Verification items for the finished model (mm, model axes). Face numbers are marked on the shaded views. Give positions to 0.01 mm unless a question says otherwise; leave off trailing zeros. Write each loop counter-clockwise with the first axis right and the second up, starting at its lowest first coordinate (ties: lowest second). Pieces come first, ordered by that corner, then holes. Notation, with made-up numbers: (16.25, 54) - (47.25, 54) arc R11 cw to (47.25, 63) - close; hole circle Ø3 at (-29.75, 48.25). An arc over 180 degrees is marked (long way). Answer as a JSON object with one key per item and string values. Group by question number.
Item 1: Sectioned sample at B-B, the plane x = 670. Record the boundary of the cut face in (y, z).
Item 2: Draft check along X on the marked faces 1 and 2. Enter one of: +X half, -X half, draft (parallel to the pull), parting line (faces both ways), or undercut.
Item 3: Scan lines: line 1 along Y through (x, z) = (808.5, 72.5); line 2 along X through (y, z) = (497, 73); line 3 along Z through (x, y) = (926.5, 1291.5). Record each from-to range of solid material in increasing order. Write a range as [from, to].
Item 4: Sectioned sample at A-A, the plane z = 366. Record the boundary of the cut face in (x, y).
Item 5: Sectioned sample at C-C, the plane y = 947.5. Record the boundary of the cut face in (x, z), and give its area (3 significant figures).
Item 6: Go/stop test with a flat-tipped pin: pin 1 (1 mm diameter, centred on x = 163.5, y = 325, fed in from -Z). Record where the tip stops, or that it passes through.
Item 7: Sectioned sample at D-D, the plane z = 78. Record the boundary of the cut face in (x, y), and give its area (3 significant figures).
```python
from build123d import *

# Parameters (mm, degrees)
F0_W      = 965.2
F0_H      = 552.45
F1_DEPTH  = 1651
F2_W      = 863.6
F2_H      = 50.8
F2_H_2    = 400.05
F3_DEPTH  = 1651
F4_W      = 1549.4
F4_H      = 50.434645
F4_H_2    = 400.415355
F5_DEPTH  = 965.2
F6_W      = 863.6
F6_H      = 749.3
F7_DEPTH  = 508
F8_W      = 85.725
F8_H      = 107.95
F9_DEPTH  = 6.35
F10_W     = 1651
F10_H     = 6.35
F11_DEPTH = 965.2


with BuildPart() as f1:
    # F0 (on Front) → F1 (new body)
    with BuildSketch(Plane.XZ):
        with Locations((482.6, 276.225)):
            Rectangle(F0_W, F0_H)
    extrude(amount=-F1_DEPTH)

    # F2 (on face) → F3 (cut, through all)
    with BuildSketch(Plane.XZ):
        with Locations((482.6, 25.4)):
            Rectangle(F2_W, F2_H)
        with Locations((482.6, 301.625)):
            Rectangle(F2_W, F2_H_2)
    extrude(amount=-F3_DEPTH, mode=Mode.SUBTRACT)

    # F4 (on face) → F5 (cut, through all)
    with BuildSketch(Plane.YZ.offset(965.2)):
        with Locations((825.5, 25.217322)):
            Rectangle(F4_W, F4_H)
        with Locations((825.5, 301.442322)):
            Rectangle(F4_W, F4_H_2)
    extrude(amount=-F5_DEPTH, mode=Mode.SUBTRACT)

    # F6 (on face) → F7 (cut)
    with BuildSketch(Plane.XY.offset(552.45)):
        with Locations((482.6, 425.45)):
            Rectangle(F6_W, F6_H)
        with Locations((482.6, 1225.55)):
            Rectangle(F6_W, F6_H)
    extrude(amount=-F7_DEPTH, mode=Mode.SUBTRACT)

    # F8 (on face) → F9 (join)
    with BuildSketch(Plane(origin=(0, 0, 0), x_dir=(1, 0, 0), z_dir=(0, 0, -1))):
        with Locations((922.3375, -1597.025)):
            Rectangle(F8_W, F8_H)
        with Locations((42.8625, -1597.025)):
            Rectangle(F8_W, F8_H)
        with Locations((922.3375, -53.975)):
            Rectangle(F8_W, F8_H)
        with Locations((42.8625, -53.975)):
            Rectangle(F8_W, F8_H)
    extrude(amount=F9_DEPTH)

    # F10 (on face) → F11 (join)
    with BuildSketch(Plane.YZ.offset(965.2)):
        with Locations((825.5, 555.625)):
            Rectangle(F10_W, F10_H)
    extrude(amount=-F11_DEPTH)


solid = f1.part
```
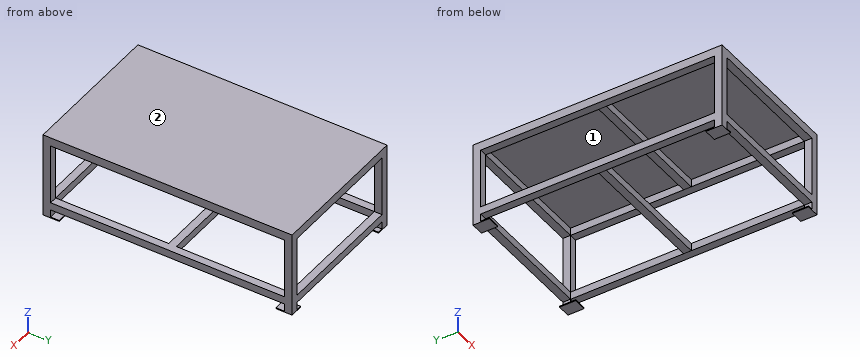
Geometry check:
{
 "1": {"outline": "(0, 50.8) - (50.8, 50.8) - (50.8, 101.6) - (0, 101.6) - close; (0, 501.65) - (50.8, 501.65) - (50.8, 552.45) - (800.1, 552.45) - (800.1, 501.65) - (850.9, 501.65) - (850.9, 552.45) - (1600.2, 552.45) - (1600.2, 501.65) - (1651, 501.65) - (1651, 558.8) - (0, 558.8) - close; (800.1, 50.8) - (850.9, 50.8) - (850.9, 101.23) - (800.1, 101.23) - close; (1600.2, 50.8) - (1651, 50.8) - (1651, 101.6) - (1600.2, 101.6) - close"},
 "2": {"face 1": "undercut", "face 2": "draft"},
 "3": {"line 1": "[0, 50.8], [800.1, 850.9], [1600.2, 1651]", "line 2": "[0, 50.8], [914.4, 965.2]", "line 3": "[50.43, 101.23], [501.65, 558.8]"},
 "4": {"outline": "(0, 0) - (50.8, 0) - (50.8, 50.8) - (0, 50.8) - close; (0, 1600.2) - (50.8, 1600.2) - (50.8, 1651) - (0, 1651) - close; (914.4, 0) - (965.2, 0) - (965.2, 50.8) - (914.4, 50.8) - close; (914.4, 1600.2) - (965.2, 1600.2) - (965.2, 1651) - (914.4, 1651) - close"},
 "5": {"outline": "(0, 50.43) - (50.8, 50.43) - (50.8, 101.23) - (0, 101.23) - close; (0, 501.65) - (50.8, 501.65) - (50.8, 552.45) - (914.4, 552.45) - (914.4, 501.65) - (965.2, 501.65) - (965.2, 558.8) - (0, 558.8) - close; (914.4, 50.43) - (965.2, 50.43) - (965.2, 101.23) - (914.4, 101.23) - close", "area": "16,500 mm^2"},
 "6": {"pin 1": "z = 552.45"},
 "7": {"outline": "(0, 0) - (965.2, 0) - (965.2, 1651) - (0, 1651) - close; hole (50.8, 50.8) - (914.4, 50.8) - (914.4, 800.1) - (50.8, 800.1) - close; hole (50.8, 850.9) - (914.4, 850.9) - (914.4, 1600.2) - (50.8, 1600.2) - close", "area": "299,000 mm^2"}
}
